Geometry check sheet. Reference: drawing and pictorial views, mm from the part's lowest x, y, z. A direction names the side the tool comes from. Round coordinates to 2 decimals unless told otherwise and drop trailing zeros. Loops run counter-clockwise (first coordinate to the right, second up) from the corner with the lowest first, then second, coordinate; pieces in that order, holes last. Notation, with made-up numbers: M 89.25,76.5 L 127.25,76.5 A22 cw 127.25,97.5 Z; hole C 79,62.25 d2. An arc over 180 degrees is marked long. One line per question, with ' | ' between items. Start each with the question number.
(1) Tool access check on the marked faces 1 and 2. Record the directions out of +Z, -Z, +X, -X, +Y, -Y that give a thin tool (end or side, any length) a straight path to the whole face; none if there is none.
(2) Section check C-C (y = 21.5). Record the boundary of the cut face in (x, z).
(3) Section check A-A (x = 10). Record the boundary of the cut face in (y, z), and give its area (3 significant figures).
(4) Thickness scan on probe 1 along X at (y, z) = (2.65, 14.5); probe 2 along Y at (x, z) = (80, 1); probe 3 along Z at (x, y) = (38.5, 6). Record the ranges inside material, lowest first. Write a range as [from, to].
(5) Section check D-D (x = 21.5). Record the boundary of the cut face in (y, z).
(6) Go/stop test with flat-tipped pins: P1, Ø1.6, axis at x = 74, z = 1, coming from the +Y side; P2, Ø4, axis at x = 84, z = 14.5, coming from the -Y side; P3, Ø8, axis at x = 28, y = 49, coming from the -Z side; P4, Ø6, axis at x = 6, z = 14.5, coming from the +Y side. Record where each tip stops, or that it passes through.
(7) Section check B-B (z = 14.5). Record the boundary of the cut face in (x, y).
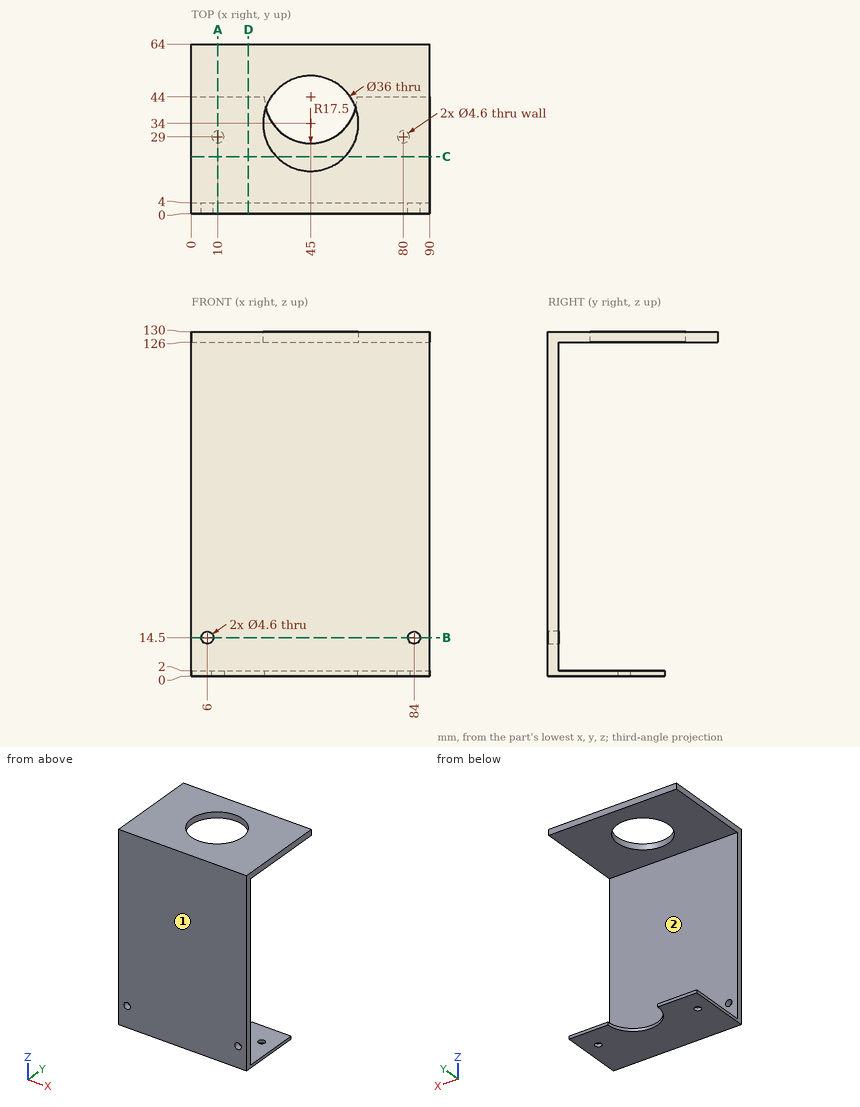
The answers:
1) face 1: +Z, -Z, +X, -X, -Y | face 2: +X, -X, +Y
2) outline: M 0,0 L 90,0 L 90,2 L 0,2 Z; M 0,126 L 32.05,126 L 32.05,130 L 0,130 Z; M 57.95,126 L 90,126 L 90,130 L 57.95,130 Z
3) outline: M 0,0 L 26.7,0 L 26.7,2 L 4,2 L 4,126 L 64,126 L 64,130 L 0,130 Z; M 31.3,0 L 44,0 L 44,2 L 31.3,2 Z | area: 831 mm²
4) probe 1: [0, 3.7], [8.3, 81.7], [86.3, 90] | probe 2: [0, 26.7], [31.3, 44] | probe 3: [0, 2], [126, 130]
5) outline: M 0,0 L 44,0 L 44,2 L 4,2 L 4,126 L 64,126 L 64,130 L 0,130 Z
6) P1: y = 44 | P2: through | P3: z = 126 | P4: y = 4
7) outline: M 0,0 L 3.7,0 L 3.7,4 L 0,4 Z; M 8.3,0 L 81.7,0 L 81.7,4 L 8.3,4 Z; M 86.3,0 L 90,0 L 90,4 L 86.3,4 Z
